Here's how the part is built. I have some questions about the finished solid (model axes, mm). Coordinates: 2 decimals unless noted, no trailing zeros. Write each loop counter-clockwise with the first axis right and the second up, starting at its lowest first coordinate (ties: lowest second). Pieces come first, ordered by that corner, then holes.
(1) Thinking about a two-plate mould opening in X: for faces 1 (the flat face through (-20, 5, 33)), 2 (the flat face through (-18, 10, 13)), 3 (the flat face through (0, 5, 23)), 4 (the cylindrical face through (-23.305, 4.93, -0.347)), which applies, released by +X, released by -X, zero draft, split by the parting line, or undercut?
(2) Imagine slicing it at A-A, the plane z = 0. List the corners of the cut face in (x, y) for me.
(3) For pin 1 Ø5 at (y, z) = (6, 34) entering from -X; pin 2 Ø4 at (x, z) = (-11, 16) entering from -Y; pin 3 Ø5 at (y, z) = (8.5, 5) entering from -X, each with a flat end and sliding along its axis, tell me the tip position at first contact or that it passes through.
(4) Imagine slicing it at D-D, the plane x = -17. List the corners of the cut face in (y, z) for me, plus the area to 3 significant figures.
(5) Please list where these lines run through material, in increasing order: probe 1 along X at (y, z) = (2.25, 36.5); probe 2 along X at (y, z) = (3.25, -3.5); probe 3 along Z at (x, y) = (-30.5, 9).
(6) Imagine slicing it at B-B, the plane y = 5.75. List the corners of the cut face in (x, z) for me, plus the area to 3 significant figures.
(7) Imagine slicing it at C-C, the plane z = 30. List the corners of the cut face in (x, y) for me.
Autodesk Inventor part; units mm, degrees
ref_plane "YZ Plane" through (0, 0, 0) normal (1, 0, 0) x (0, 1, 0)
ref_plane "XZ Plane" through (0, 0, 0) normal (0, 1, 0) x (-1, 0, 0)
ref_plane "XY Plane" through (0, 0, 0) normal (0, 0, 1) x (1, 0, 0)
sketch "Sketch1" plane through (0, 0, 0) normal (0, 1, 0) x (-1, 0, 0)
  circle A0 centre (31.197, 0) radius 7.9
  line L0 (46.197, 15) -> (0, 15)
  line L1 (0, 15) -> (0, -15)
  line L2 (0, -15) -> (46.197, -15)
  line L3 (46.197, -15) -> (46.197, 15)
  circle A1 centre (31.197, 0) radius 15
  line L4 (46.197, 15) -> (0, 15)
  line L5 (0, 15) -> (0, 42)
  line L6 (0, 42) -> (46.197, 42)
  line L7 (46.197, 42) -> (46.197, 15)
  line L8 (31.197, 15) -> (0, 42)
  point P0 (0, 0)
  point P1 (0, 0)
  point P2 (31.197, -15)
  dimension "d0" = 15.8
  dimension "d1" = 31.197
  dimension "d2" = 42
extrude "Extrusion1" add sketch "Sketch1" along normal blind 10 contours A1 L2 L1 L0 | A1 | L0 L5 L8
sketch "Sketch3" plane through (0, 10, 0) normal (0, 1, 0) x (1, 0, 0)
  circle A0 centre (-31.197, 0) radius 7.9
  circle A1 centre (-31.197, 0) radius 15.0007
  line L0 (-22.7894, 12.4231) -> (0, -3)
  line L1 (0, -42) -> (0, 15)
  line L2 (0, -3) -> (0, 15)
  line L3 (0, 15) -> (-31.1967, 15.0007)
  point P0 (0, 0)
extrude "Extrusion2" cut sketch "Sketch3" against normal blind 10 contours A1 L3 L1 L0
sketch "Sketch4" plane through (0, 10, 0) normal (0, 1, 0) x (1, 0, 0)
  line L0 (0, -42) -> (-20, -42)
  line L1 (-20, -42) -> (-20, -24)
  line L2 (-20, -24) -> (0, -24)
  line L3 (0, -24) -> (0, -42)
  point P0 (0, 0)
extrude "Extrusion3" add sketch "Sketch4" against normal blind 10
properties part number "TrubaDerzanka"
Recorded:
1. face 1: released by -X
1. face 2: zero draft
1. face 3: released by +X
1. face 4: undercut
2. outline: (-46.2, 0) - (-39.1, 0) - (-39.1, 10) - (-46.2, 10) - close; (-23.3, 0) - (-4.43, 0) - (-4.43, 10) - (-23.3, 10) - close
3. pin 1: stops at x = -20
3. pin 2: stops at y = 0
3. pin 3: stops at x = -45.99
4. outline: (0, -8.51) - (10, -8.51) - (10, 42) - (0, 42) - close
4. area: 505 mm2
5. probe 1: x = -20 to 0
5. probe 2: x = -45.78 to -38.28, -24.11 to -9.6
5. probe 3: z = -14.98 to -7.87, 7.87 to 15.6
6. outline: (-31.2, -15) - (-31.05, -15) arc R15 ccw to (-22.79, -12.42) - (0, 3) - (0, 42) - (-20, 42) - (-20, 24.69) - (-31.2, 15) arc R15 ccw to start; hole circle Ø15.8 at (-31.2, 0)
6. area: 1,450 mm2
7. outline: (-20, 0) - (0, 0) - (0, 10) - (-20, 10) - close
